```python
from build123d import *

# Parameters (mm, degrees)
F0_R     = 2.5
F1_DEPTH = 8
F3_DEPTH = 5
F5_D     = 2
F5_DEPTH = 1
F5_TIP   = 0.600860619


with BuildPart() as f1:
    # F0 (on Top) → F1 (new body)
    with BuildSketch(Plane.XY):
        Circle(F0_R)
    extrude(amount=F1_DEPTH)

    # F2 (on face) → F3 (cut)
    with BuildSketch(Plane.XY.offset(8)):
        Polygon((1.5, -0.8660254038), (1.5, 0.8660254038), (0, 1.7320508076), (-1.5, 0.8660254038), (-1.5, -0.8660254038), (0, -1.7320508076), align=None)
    extrude(amount=-F3_DEPTH, mode=Mode.SUBTRACT)

    # F5
    with Locations(Plane(origin=(0, 0, 0), x_dir=(1, 0, 0), z_dir=(0, 0, -1))):
        with Locations((0, 0)):
            Hole(F5_D / 2, depth=F5_DEPTH)
            with Locations((0, 0, -(F5_DEPTH + F5_TIP / 2))):  # 118° drill point
                Cone(0, F5_D / 2, F5_TIP, mode=Mode.SUBTRACT)


solid = f1.part
```
The model under review builds one solid part; all positions refer to its coordinate system, in mm. A direction names the side the tool comes from. Round coordinates to 2 decimals unless told otherwise and drop trailing zeros. Write each loop counter-clockwise with the first axis right and the second up, starting at its lowest first coordinate (ties: lowest second). Pieces come first, ordered by that corner, then holes. Notation, with made-up numbers: (-0.5, 38.5) -> (52.5, 38.5) arc R4 cw to (52.5, 42.5) -> close; hole circle Ø7 at (52.25, 88.25). An arc over 180 degrees is marked (long way). Use CSV: the item, a comma, the result in double quotes.
Q1. For faces 1 (the flat face through (-1.5, 0, 6)), 2 (the flat face through (1, -1, 0)), 3 (the cylindrical face through (0.217, 0.976, 0.507)), list the 3-axis set-ups (+Z, -Z, +X, -X, +Y, -Y) from which the entire face can be reached by the end or side of a thin tool; tool diameter is ignored.
Checks:
face 1,"+Z"
face 2,"-Z, +X, -X, +Y, -Y"
face 3,"-Z"
Q2. Consider section B-B (y = -1.45). Give the boundary of the cut face in (x, z).
Checks:
outline,"(-2.04, 0) -> (2.04, 0) -> (2.04, 8) -> (0.49, 8) -> (0.49, 3) -> (-0.49, 3) -> (-0.49, 8) -> (-2.04, 8) -> close"
Q3. Consider section A-A (z = 4). Give the boundary of the cut face in (x, y).
Checks:
outline,"circle Ø5 at (0, 0); hole (-1.5, -0.87) -> (0, -1.73) -> (1.5, -0.87) -> (1.5, 0.87) -> (0, 1.73) -> (-1.5, 0.87) -> close"
Q4. Mouldability with a two-part tool opening along Y and no side actions: class faces 4 (the flat face through (0, 0, 3)), 5 (the cylindrical face through (-0.54, -2.44, 3.94)), 6 (the flat face through (2, 0, 8)) as released by +Y, released by -Y, zero draft, split by the parting line, or undercut.
Checks:
face 4,"undercut"
face 5,"split by the parting line"
face 6,"zero draft"
Q5. Consider section D-D (x = 1.3). Give the boundary of the cut face in (y, z).
Checks:
outline,"(-2.14, 0) -> (2.14, 0) -> (2.14, 8) -> (0.98, 8) -> (0.98, 3) -> (-0.98, 3) -> (-0.98, 8) -> (-2.14, 8) -> close"
Q6. To check wall thickness, follow probe 1 along Y at (x, z) = (0, 0.6); probe 2 along Z at (x, y) = (-0.3, -1.45); probe 3 along Y at (x, z) = (0.5, 6.5). State the ranges of each line that lie inside material, in increasing order. Write a range as [from, to].
Checks:
probe 1,"[-2.5, -1], [1, 2.5]"
probe 2,"[0, 3]"
probe 3,"[-2.45, -1.44], [1.44, 2.45]"
Q7. For pin 1 Ø1.5 at (x, y) = (-0.5, 0) entering from +Z; pin 2 Ø1.5 at (y, z) = (1, 2.5) entering from -X, all flat-tipped, find the tip position at first contact; note any pin that passes through.
Checks:
pin 1,"z = 3"
pin 2,"x = -2.49"
Q8. Consider section C-C (z = 2). Give the boundary of the cut face in (x, y).
Checks:
outline,"circle Ø5 at (0, 0)"
